Work out the finished part from the listing and answer in its coordinate system (mm). Coordinates: 2 decimals unless noted, no trailing zeros. Order: outer loops, then holes, each group sorted by start corner. A loop starts at its lowest first (then second) coordinate and runs counter-clockwise, first axis right, second up.
1. Determine the mould class of faces 1 (the cylindrical face through (51.79, 108.88, 43.66)), 2 (the flat face through (52, 27.032, 68)), 3 (the flat face through (50.773, 69, 68)), 4 (the cylindrical face through (51.79, 31.12, 90.21)) for opening direction Y: +Y half, -Y half, draft (parallel to the pull), parting line (faces both ways), or undercut.
2. The part is cut by section C-C, the plane y = 87. Give the vertices of the cut face in (x, z), then the cut area to 3 significant figures.
3. The part is cut by section A-A, the plane x = 51.4. Give the vertices of the cut face in (y, z).
4. The part is cut by section B-B, the plane y = 39. Give the vertices of the cut face in (x, z), then the cut area to 3 significant figures.
5. Flat-ended cylindrical pins translate along their axes: pin 1 Ø5 at (y, z) = (29.53, 45.97) entering from -X; pin 2 Ø1.9 at (y, z) = (107.53, 91.45) entering from -X. Find the tip coordinate at first contact, or state that the pin passes through.
6. Find the intervals of material crossed by probe 1 along Z at (x, y) = (51.4, 101.5); probe 2 along Z at (x, y) = (51.45, 89.5), in increasing order.
```python
from build123d import *

# Parameters (mm, degrees)
BOSS_EXTRUDE1_DEPTH = 2
SKETCH2_R           = 1.6
CUT_EXTRUDE4_DEPTH  = 2


with BuildPart() as part:
    # Sketch1 → Boss-Extrude1 (new body)
    with BuildSketch(Plane(origin=(52.773284786, 0, 0), x_dir=(0, 0, -1), z_dir=(1, 0, 0))):
        Polygon((-92.505328732, 27.032359226), (-43.473908394, 27.032359226), (-42.025138005, 110.032359226), (-93.954099121, 110.032359226), align=None)
    extrude(amount=-BOSS_EXTRUDE1_DEPTH)

    # Sketch2 → Cut-Extrude4 (cut)
    with BuildSketch(Plane(origin=(52.773284786, 0, 0), x_dir=(0, 0, -1), z_dir=(1, 0, 0))):
        with Locations((-44.525138005, 107.532359226)):
            Circle(SKETCH2_R)
        with Locations((-91.454099121, 107.532359226)):
            Circle(SKETCH2_R)
        with Locations((-45.973908394, 29.532359226)):
            Circle(SKETCH2_R)
        with Locations((-90.005328732, 29.532359226)):
            Circle(SKETCH2_R)
    extrude(amount=-CUT_EXTRUDE4_DEPTH, mode=Mode.SUBTRACT)


solid = part.part
```
Geometry says:
1. face 1: undercut
1. face 2: -Y half
1. face 3: draft
1. face 4: undercut
2. outline: (50.77, 42.43) - (52.77, 42.43) - (52.77, 93.55) - (50.77, 93.55) - close
2. area: 102 mm2
3. outline: (27.03, 43.47) - (110.03, 42.03) - (110.03, 93.95) - (27.03, 92.51) - close; hole circle Ø3.2 at (29.53, 45.97); hole circle Ø3.2 at (29.53, 90.01); hole circle Ø3.2 at (107.53, 44.53); hole circle Ø3.2 at (107.53, 91.45)
4. outline: (50.77, 43.27) - (52.77, 43.27) - (52.77, 92.71) - (50.77, 92.71) - close
4. area: 98.9 mm2
5. pin 1: stops at x = 50.77
5. pin 2: passes through
6. probe 1: z = 42.17 to 93.81
6. probe 2: z = 42.38 to 93.6
